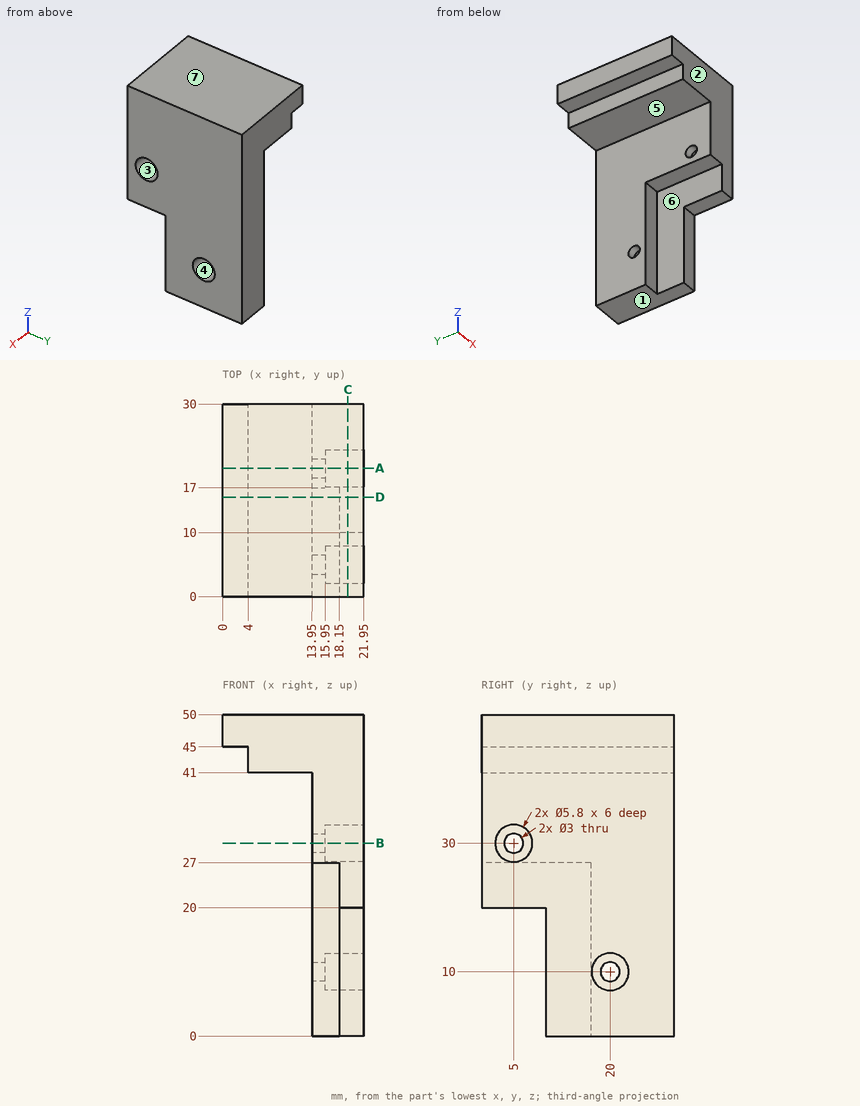
Part print with two shaded views. Sizes in mm from the minimum x, y, z corner. A direction names the side the tool comes from. Round coordinates to 2 decimals unless told otherwise and drop trailing zeros. Write each loop counter-clockwise with the first axis right and the second up, starting at its lowest first coordinate (ties: lowest second). Pieces come first, ordered by that corner, then holes. Notation, with made-up numbers: (-26, 51) -> (12, 51) arc R9 ccw to (12, 65) -> close; hole circle Ø2 at (11, 68). An arc over 180 degrees is marked (long way). Put each result on its own line as item: value.
Item 1: Slice it at B-B, the plane z = 30. Give the cut face in (x, y).
Here are the results:
outline: (13.95, 0) -> (21.95, 0) -> (21.95, 2.1) -> (15.95, 2.1) -> (15.95, 3.5) -> (13.95, 3.5) -> close; (13.95, 6.5) -> (15.95, 6.5) -> (15.95, 7.9) -> (21.95, 7.9) -> (21.95, 30) -> (13.95, 30) -> close
Item 2: Two-plate mould, pull along Z, no slides. Class the marked faces 1, 2, 3 and 4: pulls with the +Z half, pulls with the -Z half, needs draft (parallel to the pull), parting line crosses it, or undercut.
Here are the results:
face 1: pulls with the -Z half
face 2: needs draft
face 3: undercut
face 4: undercut
Item 3: Slice it at A-A, the plane y = 20. Give the cut face in (x, z), plus the area to 3 significant figures.
Here are the results:
outline: (0, 45) -> (4, 45) -> (4, 41) -> (13.95, 41) -> (13.95, 11.5) -> (15.95, 11.5) -> (15.95, 12.9) -> (21.95, 12.9) -> (21.95, 50) -> (0, 50) -> close; (13.95, 0) -> (21.95, 0) -> (21.95, 7.1) -> (15.95, 7.1) -> (15.95, 8.5) -> (13.95, 8.5) -> close
area: 469 mm^2
Item 4: Flat gauge pins, fed straight in: P1, Ø3.5, axis at y = 5, z = 30, coming from the +X side; P2, Ø2, axis at x = 2, y = 22, coming from the -Z side; P3, Ø2.5, axis at y = 5, z = 30, coming from the +X side; P4, Ø5, axis at y = 23.5, z = 41.5, coming from the -X side. Where does each tip first touch, or does it go through?
Here are the results:
P1: stops at x = 15.95
P2: stops at z = 45
P3: passes through
P4: stops at x = 4
Item 5: Slice it at C-C, the plane x = 19.5. Give the cut face in (y, z).
Here are the results:
outline: (0, 20) -> (10, 20) -> (10, 0) -> (30, 0) -> (30, 50) -> (0, 50) -> close; hole circle Ø5.8 at (5, 30); hole circle Ø5.8 at (20, 10)
Item 6: Slice it at D-D, the plane y = 15.5. Give the cut face in (x, z).
Here are the results:
outline: (0, 45) -> (4, 45) -> (4, 41) -> (13.95, 41) -> (13.95, 27) -> (18.15, 27) -> (18.15, 0) -> (21.95, 0) -> (21.95, 50) -> (0, 50) -> close
Item 7: Wall check: probe 1 along Y at (x, z) = (14.55, 10); probe 2 along Y at (x, z) = (19.85, 10); probe 3 along Z at (x, y) = (6, 2.5). Give the ranges that are in metal, low to high. Write a range as from..to.
Here are the results:
probe 1: y = 17..18.5, 21.5..30
probe 2: y = 10..17.1, 22.9..30
probe 3: z = 41..50
Item 8: Tool access for the marked faces 5, 6 and 7: list every direction of +Z, -Z, +X, -X, +Y, -Y with a clear straight run to the whole face (end or side of a thin tool).
Here are the results:
face 5: -Z, -X, +Y, -Y
face 6: -Z, -X, -Y
face 7: +Z, +X, -X, +Y, -Y
